For this review, take the finished solid that the model builds, in its own axes (mm). Face numbers are marked on the shaded views. A direction names the side the tool comes from. Give positions to 0.01 mm unless a question says otherwise; leave off trailing zeros. Write each loop counter-clockwise with the first axis right and the second up, starting at its lowest first coordinate (ties: lowest second). Pieces come first, ordered by that corner, then holes. Notation, with made-up numbers: M -11,41.25 L -3,41.25 A15 cw -3,60.25 Z; hole C 12.25,7.25 d9. An arc over 180 degrees is marked long. Write item = value, one per line.
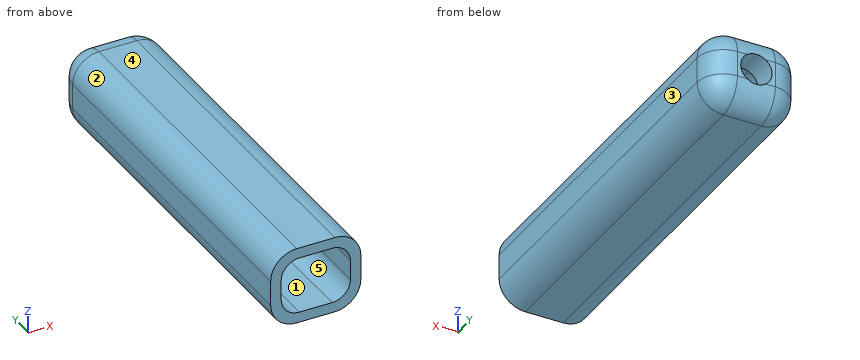
```python
from build123d import *

# Parameters (mm, degrees)
F0_W         = 17.27
F0_H         = 14.85
F0_W_2       = 13.27
F0_H_2       = 10.85
F1_DEPTH     = 75
F2_R         = 3.5
F3_R         = 5
F4_W         = 13.27
F4_H         = 10.85
F5_DEPTH     = 5
F6_R         = 3
F7_DEPTH     = 25
F8_T1_DEPTH  = 7.27
F8_T3_DEPTH  = 4.85
F8_T6_ANGLE  = 90
F8_T8_ANGLE  = 90
F8_T10_ANGLE = 90
F8_T12_ANGLE = 90


# Not quite as in the source:
# - a fillet or chamfer that OpenCascade refuses, or shapes differently, is made with other operations: its cross-section is extruded or revolved along the edge and cut away or added


with BuildPart() as f1:
    # F0 (on Front) → F1 (new body)
    with BuildSketch(Plane.XZ):
        with Locations((6.635, 5.425)):
            Rectangle(F0_W, F0_H)
        with Locations((6.635, 5.425)):
            Rectangle(F0_W_2, F0_H_2, mode=Mode.SUBTRACT)
    extrude(amount=F1_DEPTH)

    # F2
    f2_edges = [f1.edges().sort_by_distance(p)[0] for p in [
        (0, -37.5, 10.85),
        (13.27, -37.5, 0),
        (13.27, -37.5, 10.85),
        (0, -37.5, 0),
    ]]
    fillet(f2_edges, radius=F2_R)

    # F3
    f3_edges = [f1.edges().sort_by_distance(p)[0] for p in [
        (-2, -37.5, 12.85),
        (15.27, -37.5, 12.85),
        (15.27, -37.5, -2),
        (-2, -37.5, -2),
    ]]
    fillet(f3_edges, radius=F3_R)

    # F4 (on face) → F5 (join)
    with BuildSketch(Plane.XZ):
        with Locations((6.635, 5.425)):
            Rectangle(F4_W, F4_H)
    extrude(amount=F5_DEPTH)

    # F6 (on face) → F7 (cut)
    with BuildSketch(Plane.XZ):
        with Locations((6.635, 5.425)):
            Circle(F6_R)
    extrude(amount=F7_DEPTH, mode=Mode.SUBTRACT)

    # F8: fillet of radius 5 on 8 edges, made by hand

    # F8_s2 → F8_t1 (cut)
    with BuildSketch(Plane.YZ.offset(3)):
        with BuildLine():
            ThreePointArc((0, 7.85), (-1.4644660941, 11.3855339059), (-5, 12.85))
            Line((-5, 12.85), (0, 12.85))
            Line((0, 12.85), (0, 7.85))
        make_face()
        with BuildLine():
            ThreePointArc((0, 3), (-1.4644660941, -0.5355339059), (-5, -2))
            Line((-5, -2), (0, -2))
            Line((0, -2), (0, 3))
        make_face()
    extrude(amount=F8_T1_DEPTH, mode=Mode.SUBTRACT)

    # F8_s4 → F8_t3 (cut)
    with BuildSketch(Plane.XY.offset(3)):
        with BuildLine():
            ThreePointArc((3, 0), (-0.5355339059, -1.4644660941), (-2, -5))
            Line((-2, -5), (-2, 0))
            Line((-2, 0), (3, 0))
        make_face()
        with BuildLine():
            ThreePointArc((10.27, 0), (13.8055339059, -1.4644660941), (15.27, -5))
            Line((15.27, -5), (15.27, 0))
            Line((15.27, 0), (10.27, 0))
        make_face()
    extrude(amount=F8_T3_DEPTH, mode=Mode.SUBTRACT)

    # F8_s5 → F8_t6 (revolve, cut)
    with BuildSketch(Plane.XY.offset(7.85)):
        with BuildLine():
            ThreePointArc((3, 0), (-0.5355339059, -1.4644660941), (-2, -5))
            Line((-2, -5), (-2, 0))
            Line((-2, 0), (3, 0))
        make_face()
    revolve(axis=Axis((3, 0, 7.85), (0, 1, 0)), revolution_arc=F8_T6_ANGLE, mode=Mode.SUBTRACT)

    # F8_s7 → F8_t8 (revolve, cut)
    with BuildSketch(Plane.XY.offset(3)):
        with BuildLine():
            ThreePointArc((3, 0), (-0.5355339059, -1.4644660941), (-2, -5))
            Line((-2, -5), (-2, 0))
            Line((-2, 0), (3, 0))
        make_face()
    revolve(axis=Axis((3, 0, 3), (0, -1, 0)), revolution_arc=F8_T8_ANGLE, mode=Mode.SUBTRACT)

    # F8_s9 → F8_t10 (revolve, cut)
    with BuildSketch(Plane.XY.offset(7.85)):
        with BuildLine():
            ThreePointArc((10.27, 0), (13.8055339059, -1.4644660941), (15.27, -5))
            Line((15.27, -5), (15.27, 0))
            Line((15.27, 0), (10.27, 0))
        make_face()
    revolve(axis=Axis((10.27, 0, 7.85), (0, -1, 0)), revolution_arc=F8_T10_ANGLE, mode=Mode.SUBTRACT)

    # F8_s11 → F8_t12 (revolve, cut)
    with BuildSketch(Plane.YZ.offset(10.27)):
        with BuildLine():
            ThreePointArc((0, 3), (-1.4644660941, -0.5355339059), (-5, -2))
            Line((-5, -2), (0, -2))
            Line((0, -2), (0, 3))
        make_face()
    revolve(axis=Axis((10.27, 0, 3), (0, -1, 0)), revolution_arc=F8_T12_ANGLE, mode=Mode.SUBTRACT)


solid = f1.part
```
1. We need section A-A, the plane y = -37. Write out the cut boundary in (x, z), then the cut area to 3 significant figures.
Responses:
outline = M -2,3 A5 ccw 3,-2 L 10.27,-2 A5 ccw 15.27,3 L 15.27,7.85 A5 ccw 10.27,12.85 L 3,12.85 A5 ccw -2,7.85 Z; hole M 0,3.5 A3.5 ccw 3.5,0 L 9.77,0 A3.5 ccw 13.27,3.5 L 13.27,7.35 A3.5 ccw 9.77,10.85 L 3.5,10.85 A3.5 ccw 0,7.35 Z
area = 102 mm2
2. Machinability: for the marked faces 1 and 2, which of the approach directions +Z, -Z, +X, -X, +Y, -Y give a long, thin tool a straight path to every point of the face, cutting with its end or side? Answer none if there is none.
Responses:
face_1 = -Y
face_2 = +Z, -X, +Y, -Y
3. We need section C-C, the plane z = 10. Write out the cut boundary in (x, y), then the cut area to 3 significant figures.
Responses:
outline = M -1.51,-75 L 1.21,-75 L 1.21,-5 L 12.06,-5 L 12.06,-75 L 14.78,-75 L 14.78,-5 A4.51 ccw 10.27,-0.49 L 3,-0.49 A4.51 ccw -1.51,-5 Z
area = 447 mm2
4. For line 1 along Z through (x, y) = (7.5, -6); line 2 along X through (y, z) = (-54.5, 6.75); line 3 along Z through (x, y) = (2, -42.5), list the stretches that pass through material, from the lowest coordinate up. Write a range as from..to.
Responses:
line_1 = -2..0, 10.85..12.85
line_2 = -2..0, 13.27..15.27
line_3 = -1.9..0.34, 10.51..12.75
5. We need section B-B, the plane x = 12.25. Write out the cut boundary in (y, z), then the cut area to 3 significant figures.
Responses:
outline = M -75,-1.59 L -5,-1.59 A4.59 ccw -0.41,3 L -0.41,7.85 A4.59 ccw -5,12.44 L -75,12.44 L -75,9.82 L -5,9.82 L -5,1.03 L -75,1.03 Z
area = 422 mm2
6. Insertion check: P1, Ø4, axis at x = 12.5, z = 9, coming from the +Y side; P2, Ø2, axis at x = 13, y = -57, coming from the +Z side; P3, Ø4, axis at x = 10.5, y = -45, coming from the -Z side; P4, Ø5.5, axis at x = 9.5, z = 7, coming from the -Y side. Each pin has a flat end and moves straight along its axis. Give the tip position at first contact, or say it passes through.
Responses:
P1 = -0.03
P2 = 12.54
P3 = -2
P4 = -5
7. The part is to be moulded in two halves that separate along X. For the marked faces 3, 4 and 5, say which applies: +X half, -X half, draft (parallel to the pull), parting line (faces both ways), or undercut.
Responses:
face_3 = +X half
face_4 = draft
face_5 = undercut
